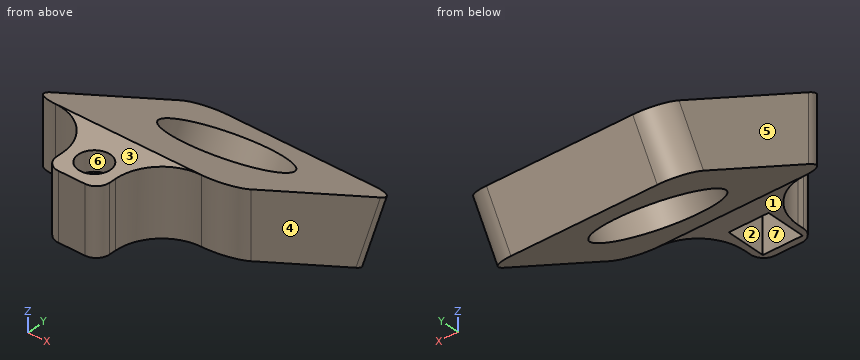
from build123d import *

# Parameters (mm, degrees)
SKETCH1_W                = 4
SKETCH1_H                = 5
BOSS_EXTRUDE1_DEPTH      = 2.5
SKETCH2_W                = 3
SKETCH2_H                = 3
CUT_EXTRUDE1_DEPTH       = 3.5
BOSS_EXTRUDE2_DEPTH      = 7.5
F_5_16_CLEARANCE_HOLE1_D = 8.4328
M2_CLEARANCE_HOLE1_D     = 2.4
FILLET1_R                = 3.5
FILLET2_R                = 2
FILLET3_R                = 1


with BuildPart() as part:
    # Sketch1 → Boss-Extrude1 (new, symmetric)
    with BuildSketch(Plane.XY):
        Rectangle(SKETCH1_W, SKETCH1_H)
    extrude(amount=BOSS_EXTRUDE1_DEPTH, both=True)

    # Sketch2 → Cut-Extrude1 (cut)
    with BuildSketch(Plane(origin=(0, 0, -2.5), x_dir=(-1, 0, 0), z_dir=(0, 0, -1))):
        with Locations((0, -0.5)):
            Rectangle(SKETCH2_W, SKETCH2_H)
    extrude(amount=-CUT_EXTRUDE1_DEPTH, mode=Mode.SUBTRACT)

    # Sketch3 → Boss-Extrude2 (add, symmetric)
    with BuildSketch(Plane(origin=(0, 0, 0), x_dir=(0, 0, -1), z_dir=(1, 0, 0))):
        Polygon((-2.5, 2.5), (6.25, 17.655444566), (10, 15.490381057), (2.5, 2.5), align=None)
    extrude(amount=BOSS_EXTRUDE2_DEPTH, both=True)

    # 5/16 Clearance Hole1 (through all)
    with Locations(Plane(origin=(0, -0.457531755, -0.792468245), x_dir=(-1, 0, 0), z_dir=(0, -0.5000000000000038, -0.8660254037844366))):
        with Locations((0, 10.915063509)):
            Hole(F_5_16_CLEARANCE_HOLE1_D / 2)

    # M2 Clearance Hole1 (through all)
    with Locations(Plane.XY.offset(2.5)):
        with Locations((0, -0.5)):
            Hole(M2_CLEARANCE_HOLE1_D / 2)

    # Fillet1
    fillet1_edges = [part.edges().sort_by_distance(p)[0] for p in [
        (-2, 2.5, 0),
        (2, 2.5, 0),
    ]]
    fillet(fillet1_edges, radius=FILLET1_R)

    # Fillet2
    fillet2_edges = [part.edges().sort_by_distance(p)[0] for p in [
        (-7.5, 16.572912811, -8.125),
        (7.5, 16.572912811, -8.125),
        (7.5, 2.5, 0),
        (-7.5, 2.5, 0),
    ]]
    fillet(fillet2_edges, radius=FILLET2_R - 0.0001)  # a hair under: the kernel refuses the full size

    # Fillet3
    fillet3_edges = [part.edges().sort_by_distance(p)[0] for p in [
        (2, -2.5, 0),
        (-2, -2.5, 0),
    ]]
    fillet(fillet3_edges, radius=FILLET3_R)


solid = part.part
Input: part model. Units: mm. Frame: model coordinates. Face numbers are marked on the shaded views. A direction names the side the tool comes from. Round coordinates to 2 decimals unless told otherwise and drop trailing zeros. Order: outer loops, then holes, each group sorted by start corner. A loop starts at its lowest first (then second) coordinate and runs counter-clockwise, first axis right, second up.
1. Pin query (flat end, axial travel): P1, Ø2.5, axis at y = -1, z = -1.5, coming from the -X side; P2, Ø4, axis at x = -5.5, z = -8, coming from the -Y side; P3, Ø2, axis at x = 3.5, z = -4.5, coming from the -Y side; P4, Ø5, axis at x = 3, y = 14, coming from the -Z side. Return the tip coordinate at first contact, or that it passes through.
The answers:
P1: stops at x = -2.23
P2: stops at y = 8.56
P3: stops at y = 4.23
P4: stops at z = -10
2. Cut plane A-A, the plane y = 0. Output: boundary loops of the cut face in (x, z).
The answers:
outline: (-2.15, -2.5) - (-1.5, -2.5) - (-1.5, 1) - (-1.09, 1) - (-1.09, 2.5) - (-2.15, 2.5) - close; (1.09, 1) - (1.5, 1) - (1.5, -2.5) - (2.15, -2.5) - (2.15, 2.5) - (1.09, 2.5) - close
3. Cut plane D-D, the plane x = -5.75. Output: boundary loops of the cut face in (y, z).
The answers:
outline: (2.52, -2.51) - (15.48, -9.99) - (17.64, -6.24) - (2.52, 2.49) - close
4. Material intervals for line 1 (X direction, y = -0.5, z = 0.25); line 2 (Y direction, x = 0, z = 2.05); line 3 (Y direction, x = 0, z = 1.65), sorted ascending.
The answers:
line 1: x = -2.04 to -1.5, 1.5 to 2.04
line 2: y = -2.5 to -1.7, 0.7 to 3.28
line 3: y = -2.5 to -1.7, 0.7 to 3.97
5. Set-up query: the marked faces 1, 2 and 3. Return all of +Z, -Z, +X, -X, +Y, -Y with unobstructed straight access to the full face (end or side cutting, diameter ignored); none if empty.
The answers:
face 1: -Z, +X, -X, -Y
face 2: -Z
face 3: +Z, +X, -X, +Y, -Y
6. Cut plane B-B, the plane x = 2.75. Output: boundary loops of the cut face in (y, z), then the cut area to 3 significant figures.
The answers:
outline: (1.17, -2.5) - (2.5, -2.5) - (6.23, -4.65) - (8.39, -0.9) - (2.5, 2.5) - (1.17, 2.5) - close; (11.76, -7.85) - (15.49, -10) - (17.66, -6.25) - (13.93, -4.1) - close
area: 49.4 mm2
7. Mould query, pull axis X, two halves, no side actions, for the marked faces 4, 5, 6 and 7. Classes: released by +X, released by -X, zero draft, split by the parting line, or undercut.
The answers:
face 4: released by +X
face 5: released by -X
face 6: undercut
face 7: undercut
8. Cut plane C-C, the plane x = 0. Output: boundary loops of the cut face in (y, z).
The answers:
outline: (-2.5, -2.5) - (-2, -2.5) - (-2, 1) - (-1.7, 1) - (-1.7, 2.5) - (-2.5, 2.5) - close; (0.7, 1) - (1, 1) - (1, -2.5) - (2.5, -2.5) - (5.34, -4.14) - (7.51, -0.39) - (2.5, 2.5) - (0.7, 2.5) - close; (12.65, -8.36) - (15.49, -10) - (17.66, -6.25) - (14.81, -4.61) - close
